Design review of the part built by this model. Coordinates are the model's own, in mm. Face numbers are marked on the shaded views. A direction names the side the tool comes from. Coordinates: 2 decimals unless noted, no trailing zeros. Order: outer loops, then holes, each group sorted by start corner. A loop starts at its lowest first (then second) coordinate and runs counter-clockwise, first axis right, second up. Notation, with made-up numbers: (70, 83) - (129, 83) arc R14 cw to (129, 93) - close; hole circle Ø2 at (-28.75, -29). An arc over 180 degrees is marked (long way). Write each question's results on one line, items separated by ' | '. Start each with the question number.
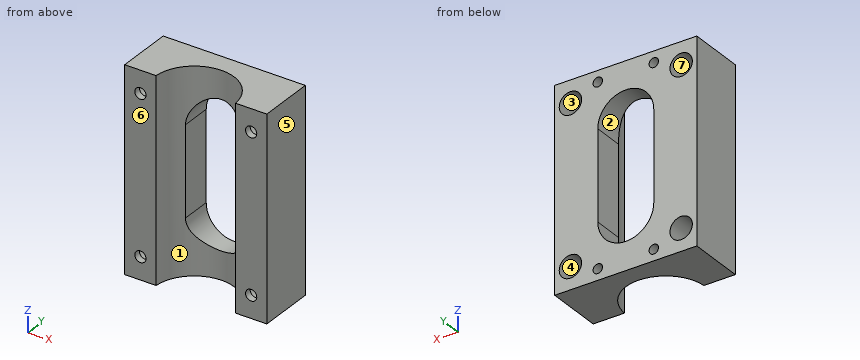
```python
from build123d import *

# Parameters (mm, degrees)
BOSS_EXTRUDE1_DEPTH             = 90
BOSS_EXTRUDE2_START             = -90
BOSS_EXTRUDE2_DEPTH             = 90
F_5_0MM_CLEARANCE_DOWEL_HOLE1_D = 5
CUT_EXTRUDE1_REACH              = 101.384
SKETCH4_R                       = 5
CUT_EXTRUDE3_DEPTH              = 101.573977748
CUT_EXTRUDE4_REACH              = 100.691
TAP_DRILL_FOR_M5X0_8_TAP1_D     = 4.2
TAP_DRILL_FOR_M5X0_8_TAP1_DEPTH = 8
TAP_DRILL_FOR_M5X0_8_TAP1_TIP   = 1.2618073


with BuildPart() as part:
    # Sketch1 → Boss-Extrude1 (new body)
    with BuildSketch(Plane.XY):
        with BuildLine():
            Line((-31.734248061, 1), (-17.721808598, 1))
            ThreePointArc((-17.721808598, 1), (0, 17.75), (17.721808598, 1))
            Line((17.721808598, 1), (31.734248061, 1))
            ThreePointArc((31.734248061, 1), (0, 31.75), (-31.734248061, 1))
        make_face()
    extrude(amount=BOSS_EXTRUDE1_DEPTH)

    # Sketch12 → Boss-Extrude2 (add)
    with BuildSketch(Plane.XY.offset(90).offset(BOSS_EXTRUDE2_START)):
        with BuildLine():
            Line((31.734248061, 31.75), (0, 31.75))
            ThreePointArc((0, 31.75), (22.094258304, 22.801452805), (31.734248061, 1))
            Line((31.734248061, 1), (31.734248061, 31.75))
        make_face()
        with BuildLine():
            Line((-31.734248061, 31.75), (-31.734248061, 1))
            ThreePointArc((-31.734248061, 1), (-22.094258304, 22.801452805), (0, 31.75))
            Line((0, 31.75), (-31.734248061, 31.75))
        make_face()
    extrude(amount=BOSS_EXTRUDE2_DEPTH)

    # Ø5.0mm Clearance Dowel Hole1 (through all)
    with Locations(Plane(origin=(-24.72802833, 1, 80), x_dir=(0, 0, -1), z_dir=(0, -1, 0))):
        with Locations((0, 0), (70, 0), (0, 49.45605666), (70, 49.45605666)):
            Hole(F_5_0MM_CLEARANCE_DOWEL_HOLE1_D / 2)

    # Sketch4 → Cut-Extrude1 (cut, up to next)
    with BuildSketch(Plane(origin=(0, 4, 0), x_dir=(-1, 0, 0), z_dir=(0, -1, 0)), mode=Mode.PRIVATE) as cut_extrude1_sk1:
        with Locations(Location((24.72802833, -80, 0), (0, 0, 90))):
            Circle(SKETCH4_R)
    cut_extrude1_tool1 = extrude(cut_extrude1_sk1.sketch, amount=-CUT_EXTRUDE1_REACH, mode=Mode.PRIVATE) & part.part
    # Sketch4 → Cut-Extrude1 (cut, up to next)
    with BuildSketch(Plane(origin=(0, 4, 0), x_dir=(-1, 0, 0), z_dir=(0, -1, 0)), mode=Mode.PRIVATE) as cut_extrude1_sk2:
        with Locations(Location((24.72802833, -10, 0), (0, 0, 90))):
            Circle(SKETCH4_R)
    cut_extrude1_tool2 = extrude(cut_extrude1_sk2.sketch, amount=-CUT_EXTRUDE1_REACH, mode=Mode.PRIVATE) & part.part
    # Sketch4 → Cut-Extrude1 (cut, up to next)
    with BuildSketch(Plane(origin=(0, 4, 0), x_dir=(-1, 0, 0), z_dir=(0, -1, 0)), mode=Mode.PRIVATE) as cut_extrude1_sk3:
        with Locations(Location((-24.72802833, -10, 0), (0, 0, 90))):
            Circle(SKETCH4_R)
    cut_extrude1_tool3 = extrude(cut_extrude1_sk3.sketch, amount=-CUT_EXTRUDE1_REACH, mode=Mode.PRIVATE) & part.part
    # Sketch4 → Cut-Extrude1 (cut, up to next)
    with BuildSketch(Plane(origin=(0, 4, 0), x_dir=(-1, 0, 0), z_dir=(0, -1, 0)), mode=Mode.PRIVATE) as cut_extrude1_sk4:
        with Locations(Location((-24.72802833, -80, 0), (0, 0, 90))):
            Circle(SKETCH4_R)
    cut_extrude1_tool4 = extrude(cut_extrude1_sk4.sketch, amount=-CUT_EXTRUDE1_REACH, mode=Mode.PRIVATE) & part.part
    add(cut_extrude1_tool1.solids().sort_by_distance((-24.728028, 4, 80))[0], mode=Mode.SUBTRACT)
    add(cut_extrude1_tool2.solids().sort_by_distance((-24.728028, 4, 10))[0], mode=Mode.SUBTRACT)
    add(cut_extrude1_tool3.solids().sort_by_distance((24.728028, 4, 10))[0], mode=Mode.SUBTRACT)
    add(cut_extrude1_tool4.solids().sort_by_distance((24.728028, 4, 80))[0], mode=Mode.SUBTRACT)

    # Sketch8 → Cut-Extrude3 (cut, through all)
    with BuildSketch(Plane.XY.offset(90)):
        with BuildLine():
            Line((-31.734248061, 26.154588508), (-18, 26.154588508))
            ThreePointArc((-18, 26.154588508), (-9.424816043, 30.318894151), (0, 31.75))
            Line((0, 31.75), (-31.734248061, 31.75))
            Line((-31.734248061, 31.75), (-31.734248061, 26.154588508))
        make_face()
        with BuildLine():
            Line((18, 26.154588508), (-18, 26.154588508))
            ThreePointArc((-18, 26.154588508), (0, 31.75), (18, 26.154588508))
        make_face()
        with BuildLine():
            ThreePointArc((0, 31.75), (9.424816043, 30.318894151), (18, 26.154588508))
            Line((18, 26.154588508), (31.734248061, 26.154588508))
            Line((31.734248061, 26.154588508), (31.734248061, 31.75))
            Line((31.734248061, 31.75), (0, 31.75))
        make_face()
    extrude(amount=-CUT_EXTRUDE3_DEPTH, mode=Mode.SUBTRACT)

    # Sketch9 → Cut-Extrude4 (cut, up to next)
    with BuildSketch(Plane.XZ.offset(-1), mode=Mode.PRIVATE) as cut_extrude4_sk1:
        with BuildLine():
            Line((-12.5, 25), (-12.5, 65))
            ThreePointArc((-12.5, 65), (0, 77.5), (12.5, 65))
            Line((12.5, 65), (12.5, 25))
            ThreePointArc((12.5, 25), (0, 12.5), (-12.5, 25))
        make_face()
    cut_extrude4_tool1 = extrude(cut_extrude4_sk1.sketch, amount=-CUT_EXTRUDE4_REACH, mode=Mode.PRIVATE) & part.part
    add(cut_extrude4_tool1.solids().sort_by_distance((0, 1, 45))[0], mode=Mode.SUBTRACT)

    # Tap Drill for M5x0.8 Tap1
    with Locations(Plane(origin=(-12.5, 26.154588508, 5), x_dir=(0, 0, 1), z_dir=(0, 1, 0))):
        with Locations((0, 0), (0, 25), (80, 25), (80, 0)):
            Hole(TAP_DRILL_FOR_M5X0_8_TAP1_D / 2, depth=TAP_DRILL_FOR_M5X0_8_TAP1_DEPTH)
            with Locations((0, 0, -(TAP_DRILL_FOR_M5X0_8_TAP1_DEPTH + TAP_DRILL_FOR_M5X0_8_TAP1_TIP / 2))):  # 118° drill point
                Cone(0, TAP_DRILL_FOR_M5X0_8_TAP1_D / 2, TAP_DRILL_FOR_M5X0_8_TAP1_TIP, mode=Mode.SUBTRACT)


solid = part.part
```
(1) Take a section at C-C (y = 15.75). State the section outline as (x, z) points, plus the area to 3 significant figures.
(2) Take a section at A-A (z = 80). State the section outline as (x, y) points.
(3) Take a section at D-D (z = 34.5). State the section outline as (x, y) points, plus the area to 3 significant figures.
(4) Take a section at B-B (x = 0). State the section outline as (y, z) points.
(5) Clearance check with flat-ended pins moving along their axes: pin 1 (3 mm diameter, centred on x = -25, z = 81, fed in from +Y); pin 2 (3.5 mm diameter, centred on x = 12.5, z = 85, fed in from -Y). State where each tip first meets the part, or that it passes through.
(6) To check wall thickness, follow line 1 along X through (y, z) = (20, 10); line 2 along X through (y, z) = (2.8, 80); line 3 along X through (y, z) = (18, 58). State the ranges of each line that lie inside material, in increasing order. Write a range as [from, to].
(7) Mouldability with a two-part tool opening along X and no side actions: class the marked faces 4, 5, 6 and 7 as +X half, -X half, draft (parallel to the pull), parting line (faces both ways), or undercut.
(8) Tool access review of the marked faces 1, 2 and 3: name each direction out of +Z, -Z, +X, -X, +Y, -Y from which nothing blocks a thin tool from reaching the whole face with its end or side.
Worked out:
1) outline: (-31.73, 0) - (-8.19, 0) - (-8.19, 15.55) arc R12.5 cw to (-12.5, 25) - (-12.5, 65) arc R12.5 cw to (-8.19, 74.45) - (-8.19, 90) - (-31.73, 90) - close; (8.19, 0) - (31.73, 0) - (31.73, 90) - (8.19, 90) - (8.19, 74.45) arc R12.5 cw to (12.5, 65) - (12.5, 25) arc R12.5 cw to (8.19, 15.55) - close; hole circle Ø10 at (-24.73, 10); hole circle Ø10 at (-24.73, 80); hole circle Ø10 at (24.73, 10); hole circle Ø10 at (24.73, 80) | area: 3,470 mm^2
2) outline: (-31.73, 1) - (-27.23, 1) - (-27.23, 4) - (-29.73, 4) - (-29.73, 26.15) - (-31.73, 26.15) - close; (-22.23, 1) - (-17.72, 1) arc R17.75 cw to (17.72, 1) - (22.23, 1) - (22.23, 4) - (19.73, 4) - (19.73, 26.15) - (-19.73, 26.15) - (-19.73, 4) - (-22.23, 4) - close; (27.23, 1) - (31.73, 1) - (31.73, 26.15) - (29.73, 26.15) - (29.73, 4) - (27.23, 4) - close
3) outline: (-31.73, 1) - (-17.72, 1) arc R17.75 cw to (-12.5, 12.6) - (-12.5, 26.15) - (-31.73, 26.15) - close; (12.5, 12.6) arc R17.75 cw to (17.72, 1) - (31.73, 1) - (31.73, 26.15) - (12.5, 26.15) - close | area: 887 mm^2
4) outline: (17.75, 0) - (26.15, 0) - (26.15, 12.5) - (17.75, 12.5) - close; (17.75, 77.5) - (26.15, 77.5) - (26.15, 90) - (17.75, 90) - close
5) pin 1: y = 4 | pin 2: y = 10.58
6) line 1: [-31.73, -29.73], [-19.73, 19.73], [29.73, 31.73] | line 2: [-31.73, -27.23], [-22.23, -17.53], [17.53, 22.23], [27.23, 31.73] | line 3: [-31.73, -12.5], [12.5, 31.73]
7) face 4: undercut | face 5: +X half | face 6: draft | face 7: undercut
8) face 1: +Z, -Z, -Y | face 2: +Y, -Y | face 3: +Y
